Can you work these out from the model? Positions are in its coordinate system, mm. Coordinates: 2 decimals unless noted, no trailing zeros. Loops run counter-clockwise (first coordinate to the right, second up) from the corner with the lowest first, then second, coordinate; pieces in that order, holes last.
Autodesk Inventor part; units mm, degrees
ref_plane "YZ Plane" through (0, 0, 0) normal (1, 0, 0) x (0, 1, 0)
ref_plane "XZ Plane" through (0, 0, 0) normal (0, 1, 0) x (-1, 0, 0)
ref_plane "XY Plane" through (0, 0, 0) normal (0, 0, 1) x (1, 0, 0)
sketch "Sketch1" plane through (0, 0, 0) normal (0, 0, 1) x (1, 0, 0)
  arc A0 (4.9396, -4.0821) -> (-3.0171, -14.3627) centre (0.9613, -9.2224) ccw
  arc A1 (13.9722, -27.5116) -> (21.9289, -17.231) centre (17.9505, -22.3713) ccw
  line L0 (4.9396, -4.0821) -> (21.9289, -17.231)
  line L1 (-3.0171, -14.3627) -> (13.9722, -27.5116)
  point P0 (0, 0)
  dimension "d0" = 13
  dimension "d1" = 13
extrude "Extrusion1" add sketch "Sketch1" along normal mid plane 2.2625
hole "Hole1" at (0.9613, -9.2224, 0) at (17.9505, -22.3713, 0) direction (0, 0, 1) diameter 5.159 end through all both
properties part number "smallthing"
Item 1: Suppose I cut it at B-B, the plane y = -21. Please give me the cut outline in (x, z), plus the area to 3 significant figures.
Results are:
outline: (5.56, -1.13) - (15.77, -1.13) - (15.77, 1.13) - (5.56, 1.13) - close; (20.14, -1.13) - (24.3, -1.13) - (24.3, 1.13) - (20.14, 1.13) - close
area: 32.5 mm2
Item 2: I need wall thicknesses on line 1 along X through (y, z) = (-20.5, -0.15); line 2 along X through (y, z) = (-23.75, 0.1); line 3 along Y through (x, z) = (1.25, -0.9). Which ranges of each line are inside material? Lowest first, please.
Results are:
line 1: x = 4.91 to 16.18, 19.73 to 24.18
line 2: x = 9.11 to 15.77, 20.13 to 24.3
line 3: y = -17.67 to -11.79, -6.66 to -2.73
Item 3: I'm going to push flat-ended pins straight in: P1, Ø8.5, axis at x = 17.95, y = -22.37, coming from the +Z side; P2, Ø4.5, axis at x = 0.96, y = -9.22, coming from the -Z side. Where does each tip first touch, or does it pass through?
Results are:
P1: stops at z = 1.13
P2: passes through
Item 4: We'd pull the mould along Y, two halves only. Please class faces 1 (the face through (0.85, -11.8, 0.02)), 2 (the face through (23.177, -26.236, -0.016)), 3 (the face through (9, -16, 1.131)): +Y half, -Y half, draft (parallel to the pull), parting line (faces both ways), or undercut.
Results are:
face 1: undercut
face 2: parting line
face 3: draft
Item 5: Suppose I cut it at C-C, the plane z = -0.1. Please give me the cut outline in (x, y), plus the area to 3 significant figures.
Results are:
outline: (-3.02, -14.36) - (13.97, -27.51) arc R6.5 ccw to (21.93, -17.23) - (4.94, -4.08) arc R6.5 ccw to start; hole circle Ø5.16 at (0.96, -9.22); hole circle Ø5.16 at (17.95, -22.37)
area: 370 mm2
Item 6: Suppose I cut it at D-D, the plane x = -3.5. Please give me the cut outline in (y, z).
Results are:
outline: (-13.95, -1.13) - (-4.5, -1.13) - (-4.5, 1.13) - (-13.95, 1.13) - close
Item 7: Suppose I cut it at A-A, the plane x = 15.75. Please give me the cut outline in (y, z), plus the area to 3 significant figures.
Results are:
outline: (-28.49, -1.13) - (-23.72, -1.13) - (-23.72, 1.13) - (-28.49, 1.13) - close; (-21.03, -1.13) - (-12.45, -1.13) - (-12.45, 1.13) - (-21.03, 1.13) - close
area: 30.2 mm2
